```python
from build123d import *

# Parameters (mm, degrees)
BOSS_EXTRUDE1_DEPTH      = 35.687
BOSS_EXTRUDE1_DEPTH_BACK = 35.687
CUT_EXTRUDE1_DEPTH       = 88.202032482
CUT_EXTRUDE1_DEPTH_BACK  = 88.202032482
CUT_EXTRUDE2_DEPTH       = 88.202032482
CUT_EXTRUDE2_DEPTH_BACK  = 88.202032482
SKETCH6_R                = 4.1656
SKETCH7_R                = 4.1656
CUT_EXTRUDE3_DEPTH       = 88.202032482


with BuildPart() as part:
    # Sketch4 → Boss-Extrude1 (new, two sides: drawn at the far end of the back side and taken through both)
    with BuildSketch(Plane.XY.offset(-BOSS_EXTRUDE1_DEPTH_BACK)):
        with BuildLine():
            Line((-38.1, 38.1), (-38.1, -38.1))
            Line((-38.1, -38.1), (38.1, -38.1))
            ThreePointArc((38.1, -38.1), (36.240128061, -33.609871939), (31.75, -31.75))
            Line((31.75, -31.75), (-23.8252, -31.75))
            ThreePointArc((-23.8252, -31.75), (-29.42887982, -29.42887982), (-31.75, -23.8252))
            Line((-31.75, -23.8252), (-31.75, 31.75))
            ThreePointArc((-31.75, 31.75), (-33.609871939, 36.240128061), (-38.1, 38.1))
        make_face()
    extrude(amount=BOSS_EXTRUDE1_DEPTH + BOSS_EXTRUDE1_DEPTH_BACK)

    # Sketch5 → Cut-Extrude1 (cut, two sides: drawn at the far end of the back side and taken through both)
    with BuildSketch(Plane(origin=(-31.75, 0, 0), x_dir=(0, 0, -1), z_dir=(1, 0, 0)).offset(-CUT_EXTRUDE1_DEPTH_BACK)):
        Polygon((-35.687, -23.8252), (-16.637, 38.1), (-35.687, 38.1), align=None)
        Polygon((35.687, 38.1), (16.637, 38.1), (35.687, -23.8252), align=None)
    extrude(amount=CUT_EXTRUDE1_DEPTH + CUT_EXTRUDE1_DEPTH_BACK, mode=Mode.SUBTRACT)

    # Sketch6 → Cut-Extrude2 (cut, two sides: drawn at the far end of the back side and taken through both)
    with BuildSketch(Plane(origin=(-31.75, 0, 0), x_dir=(0, 0, -1), z_dir=(1, 0, 0)).offset(-CUT_EXTRUDE2_DEPTH_BACK)):
        with Locations(Location((0, 19.05, 0), (0, 0, 90))):
            Circle(SKETCH6_R)
        with Locations(Location((0, -19.05, 0), (0, 0, 90))):
            Circle(SKETCH6_R)
    extrude(amount=CUT_EXTRUDE2_DEPTH + CUT_EXTRUDE2_DEPTH_BACK, mode=Mode.SUBTRACT)

    # Sketch7 → Cut-Extrude3 (cut, through all)
    with BuildSketch(Plane(origin=(0, -31.75, 0), x_dir=(1, 0, 0), z_dir=(0, 1, 0))):
        with Locations(Location((-19.05, 19.05, 0), (0, 0, 180))):
            Circle(SKETCH7_R)
        with Locations((19.05, 19.05)):
            Circle(SKETCH7_R)
        with Locations(Location((19.05, -19.05, 0), (0, 0, 180))):
            Circle(SKETCH7_R)
        with Locations((-19.05, -19.05)):
            Circle(SKETCH7_R)
    extrude(amount=-CUT_EXTRUDE3_DEPTH, mode=Mode.SUBTRACT)


solid = part.part
```
The model under review builds one solid part; all positions refer to its coordinate system, in mm. A direction names the side the tool comes from. Round coordinates to 2 decimals unless told otherwise and drop trailing zeros. Order: outer loops, then holes, each group sorted by start corner. A loop starts at its lowest first (then second) coordinate and runs counter-clockwise, first axis right, second up.
(1) Take a section at B-B, the plane z = 0. State the section outline as (x, y) points, plus the area to 3 significant figures.
Working result:
outline: (-38.1, -38.1) - (38.1, -38.1) arc R6.35 ccw to (31.75, -31.75) - (-23.83, -31.75) arc R7.92 cw to (-31.75, -23.83) - (-31.75, -23.22) - (-38.1, -23.22) - close; (-38.1, -14.88) - (-31.75, -14.88) - (-31.75, 14.88) - (-38.1, 14.88) - close; (-38.1, 23.22) - (-31.75, 23.22) - (-31.75, 31.75) arc R6.35 ccw to (-38.1, 38.1) - close
area: 818 mm2
(2) Take a section at D-D, the plane z = -11.5. State the section outline as (x, y) points.
Working result:
outline: (-38.1, -38.1) - (38.1, -38.1) arc R6.35 ccw to (31.75, -31.75) - (-23.83, -31.75) arc R7.92 cw to (-31.75, -23.83) - (-31.75, 31.75) arc R6.35 ccw to (-38.1, 38.1) - close
(3) Wall thickness on L1, parallel to Z at x = 19.05, y = -36.5; L2, parallel to Y at x = -34, z = 0; L3, parallel to Y at x = -22, z = 7: over which ranges is each line inside the solid? List them lowest first.
Working result:
L1: z = -35.69 to -23.22, -14.88 to 14.88, 23.22 to 35.69
L2: y = -38.1 to -23.22, -14.88 to 14.88, 23.22 to 36.6
L3: y = -38.1 to -31.75
(4) Tool access review of faces 5 (the face through (-31.75, 4, 0)), 6 (the face through (-19.59, -34.88, 14.92)): name each direction out of +Z, -Z, +X, -X, +Y, -Y from which nothing blocks a thin tool from reaching the whole face with its end or side.
Working result:
face 5: +Z, -Z, +X, +Y
face 6: +Y, -Y
(5) Take a section at C-C, the plane y = 19.05. State the section outline as (x, z) points.
Working result:
outline: (-38.1, -22.5) - (-31.75, -22.5) - (-31.75, -4.17) - (-38.1, -4.17) - close; (-38.1, 4.17) - (-31.75, 4.17) - (-31.75, 22.5) - (-38.1, 22.5) - close
(6) For P1, Ø2, axis at y = 19, z = 11, coming from the +X side; P2, Ø1, axis at x = -2.5, z = 11, coming from the +Y side; P3, Ø11, axis at x = -19.05, z = -19.05, coming from the +Y side, all flat-tipped, find the tip position at first contact; note any pin that passes through.
Working result:
P1: stops at x = -31.75
P2: stops at y = -31.75
P3: stops at y = -31.72
(7) Take a section at A-A, the plane x = -19.05. State the section outline as (y, z) points, plus the area to 3 significant figures.
Working result:
outline: (-38.1, -35.69) - (-31.75, -35.69) - (-31.75, -23.22) - (-38.1, -23.22) - close; (-38.1, -14.88) - (-31.75, -14.88) - (-31.75, 14.88) - (-38.1, 14.88) - close; (-38.1, 23.22) - (-31.75, 23.22) - (-31.75, 35.69) - (-38.1, 35.69) - close
area: 347 mm2
(8) Mouldability with a two-part tool opening along X and no side actions: class faces 1 (the face through (-33.56, 36.19, -0.26)), 2 (the face through (-38.1, -8, 0)), 3 (the face through (-1, -34, -35.687)), 4 (the face through (-18.51, -34.88, -14.92)) as released by +X, released by -X, zero draft, split by the parting line, or undercut.
Working result:
face 1: released by +X
face 2: released by -X
face 3: zero draft
face 4: undercut
